from build123d import *

# Parameters (mm, degrees)
SKETCH1_W           = 133.35
SKETCH1_H           = 139.7
BOSS_EXTRUDE1_DEPTH = 25.4
SKETCH2_W           = 50.8
SKETCH2_H           = 114.3
BOSS_EXTRUDE2_DEPTH = 12.7
SKETCH3_R           = 3.175
BOSS_EXTRUDE3_DEPTH = 38.1
SKETCH4_R           = 3.175
BOSS_EXTRUDE4_DEPTH = 38.1
SKETCH5_R           = 3.175
BOSS_EXTRUDE5_DEPTH = 25.4
SKETCH6_R           = 3.175
BOSS_EXTRUDE6_DEPTH = 25.4


with BuildPart() as part:
    # Sketch1 → Boss-Extrude1 (new body)
    with BuildSketch(Plane(origin=(0, 0, 0), x_dir=(1, 0, 0), z_dir=(0, 1, 0))):
        with Locations((66.675, 42.031328285)):
            Rectangle(SKETCH1_W, SKETCH1_H)
    extrude(amount=BOSS_EXTRUDE1_DEPTH)

    # Sketch2 → Boss-Extrude2 (add)
    with BuildSketch(Plane(origin=(0, 0, 0), x_dir=(-1, 0, 0), z_dir=(0, -1, 0))):
        with Locations((-107.95, 42.031328285)):
            Rectangle(SKETCH2_W, SKETCH2_H)
    extrude(amount=BOSS_EXTRUDE2_DEPTH)

    # Sketch3 → Boss-Extrude3 (add)
    with BuildSketch(Plane(origin=(0, 0, 0), x_dir=(-1, 0, 0), z_dir=(0, -1, 0))):
        with Locations((-3.175, 96.641328285)):
            Circle(SKETCH3_R)
    extrude(amount=BOSS_EXTRUDE3_DEPTH)

    # Sketch4 → Boss-Extrude4 (add)
    with BuildSketch(Plane(origin=(0, 0, 0), x_dir=(-1, 0, 0), z_dir=(0, -1, 0))):
        with Locations((-3.175, -12.578671715)):
            Circle(SKETCH4_R)
    extrude(amount=BOSS_EXTRUDE4_DEPTH)

    # Sketch5 → Boss-Extrude5 (add)
    with BuildSketch(Plane(origin=(0, -12.7, 0), x_dir=(-1, 0, 0), z_dir=(0, -1, 0))):
        with Locations((-130.175, 96.641328285)):
            Circle(SKETCH5_R)
    extrude(amount=BOSS_EXTRUDE5_DEPTH)

    # Sketch6 → Boss-Extrude6 (add)
    with BuildSketch(Plane(origin=(0, -12.7, 0), x_dir=(-1, 0, 0), z_dir=(0, -1, 0))):
        with Locations((-130.175, -12.578671715)):
            Circle(SKETCH6_R)
    extrude(amount=BOSS_EXTRUDE6_DEPTH)


solid = part.part
The listing builds one solid part. Answer for the finished solid, in the listing's coordinates (mm). A direction names the side the tool comes from. Give positions to 0.01 mm unless a question says otherwise; leave off trailing zeros. Write each loop counter-clockwise with the first axis right and the second up, starting at its lowest first coordinate (ties: lowest second). Pieces come first, ordered by that corner, then holes. Notation, with made-up numbers: (28, 72.25) -> (34, 72.25) arc R19 cw to (34, 85.25) -> close; hole circle Ø11 at (-28, 14.5). An arc over 180 degrees is marked (long way). Use a Markdown table: item, result.
(1) Section A-A, the plane x = 97.5 is taken. Determine the outline of the cut face in (y, z).
Return value:
| item | result |
|---|---|
| outline | (-12.7, -99.18) -> (0, -99.18) -> (0, -111.88) -> (25.4, -111.88) -> (25.4, 27.82) -> (0, 27.82) -> (0, 15.12) -> (-12.7, 15.12) -> close |
(2) Section D-D, the plane z = -34.5 is taken. Determine the outline of the cut face in (x, y), then the cut area to 3 significant figures.
Return value:
| item | result |
|---|---|
| outline | (0, 0) -> (82.55, 0) -> (82.55, -12.7) -> (133.35, -12.7) -> (133.35, 25.4) -> (0, 25.4) -> close |
| area | 4,030 mm2 |
(3) Determine the mould class of faces 1 (the cylindrical face through (1.47, -18.78, -99.32)), 2 (the flat face through (3, -38.1, 13)), 3 (the flat face through (133.35, 6, -41)) for opening direction X: released by +X, released by -X, zero draft, split by the parting line, or undercut.
Return value:
| item | result |
|---|---|
| face 1 | undercut |
| face 2 | zero draft |
| face 3 | released by +X |
(4) For faces 4 (the cylindrical face through (1.71, -18.783, 15.395)), 5 (the flat face through (66, 13, -111.881)), determine the directions among +Z, -Z, +X, -X, +Y, -Y from which every point of the face is accessible in a straight line to the end or side of a thin tool.
Return value:
| item | result |
|---|---|
| face 4 | -Y |
| face 5 | -Z, +X, -X, +Y, -Y |
(5) Section B-B, the plane y = -7 is taken. Determine the outline of the cut face in (x, z) (3 decimals), then the cut area to 3 significant figures.
Return value:
| item | result |
|---|---|
| outline | circle Ø6.35 at (3.175, -96.641); circle Ø6.35 at (3.175, 12.579); (82.55, -99.181) -> (133.35, -99.181) -> (133.35, 15.119) -> (82.55, 15.119) -> close |
| area | 5,870 mm2 |
(6) Section C-C, the plane y = -31 is taken. Determine the outline of the cut face in (x, z) (3 decimals), then the cut area to 3 significant figures.
Return value:
| item | result |
|---|---|
| outline | circle Ø6.35 at (3.175, -96.641); circle Ø6.35 at (3.175, 12.579); circle Ø6.35 at (130.175, -96.641); circle Ø6.35 at (130.175, 12.579) |
| area | 127 mm2 |
(7) Flat-ended cylindrical pins translate along their axes: P1, Ø6.5, axis at y = -6, z = -25.5, coming from the -X side; P2, Ø6.5, axis at x = 107.5, y = -7, coming from the +Z side; P3, Ø5, axis at y = -15.5, z = 6, coming from the -X side; P4, Ø4, axis at x = 118.5, y = -7, coming from the -Z side. Find the tip coordinate at first contact, or state that the pin passes through.
Return value:
| item | result |
|---|---|
| P1 | x = 82.55 |
| P2 | z = 15.12 |
| P3 | through |
| P4 | z = -99.18 |
(8) Find the intervals of material crossed by probe 1 along X at (y, z) = (-32, 12.5); probe 2 along Y at (x, z) = (118, 4); probe 3 along X at (y, z) = (-7.5, -7), in increasing order. Write a range as from..to.
Return value:
| item | result |
|---|---|
| probe 1 | 0..6.35, 127..133.35 |
| probe 2 | -12.7..25.4 |
| probe 3 | 82.55..133.35 |
